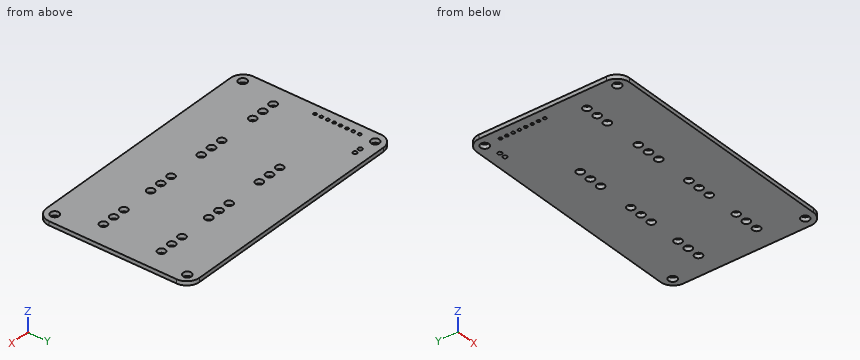
from build123d import *

# Parameters (mm, degrees)
BOSS_EXTRUDE1_DEPTH = 1.6
MULTI_LAYER_R       = 0.6
MULTI_LAYER_R_2     = 1.5
MULTI_LAYER_R_3     = 0.8
MULTI_LAYER_R_4     = 1.6500127
CUT_EXTRUDE2_DEPTH  = 1.6


with BuildPart() as part:
    # BoardOutLine → Boss-Extrude1 (new body)
    with BuildSketch(Plane.XY):
        with BuildLine():
            Line((0, -55), (0, -5))
            ThreePointArc((0, -5), (1.464466094, -1.464466094), (5, 0))
            Line((5, 0), (95, 0))
            ThreePointArc((95, 0), (98.535533906, -1.464466094), (100, -5))
            Line((100, -5), (100, -55))
            ThreePointArc((100, -55), (98.535533906, -58.535533906), (95, -60))
            Line((95, -60), (5, -60))
            ThreePointArc((5, -60), (1.464466094, -58.535533906), (0, -55))
        make_face()
    extrude(amount=BOSS_EXTRUDE1_DEPTH)

    # Multi-Layer → Cut-Extrude2 (cut)
    with BuildSketch(Plane.XY.offset(1.6)):
        with Locations((3.937007874, -25.172974346)):
            Circle(MULTI_LAYER_R)
        with Locations((3.937007874, -22.673101346)):
            Circle(MULTI_LAYER_R)
        with Locations((3.937007874, -20.172974346)):
            Circle(MULTI_LAYER_R)
        with Locations((3.937007874, -17.673101346)):
            Circle(MULTI_LAYER_R)
        with Locations((3.937007874, -15.172974346)):
            Circle(MULTI_LAYER_R)
        with Locations((3.937007874, -12.673101346)):
            Circle(MULTI_LAYER_R)
        with Locations((3.937007874, -10.172974346)):
            Circle(MULTI_LAYER_R)
        with Locations((32.974345949, -41.021082042)):
            Circle(MULTI_LAYER_R_2)
        with Locations((37.973075946, -41.021082042)):
            Circle(MULTI_LAYER_R_2)
        with Locations((42.974345949, -41.021082042)):
            Circle(MULTI_LAYER_R_2)
        with Locations((57.739395479, -41.021082042)):
            Circle(MULTI_LAYER_R_2)
        with Locations((62.738125476, -41.021082042)):
            Circle(MULTI_LAYER_R_2)
        with Locations((67.739395479, -41.021082042)):
            Circle(MULTI_LAYER_R_2)
        with Locations((80.853441707, -41.021082042)):
            Circle(MULTI_LAYER_R_2)
        with Locations((85.852171704, -41.021082042)):
            Circle(MULTI_LAYER_R_2)
        with Locations((90.853441707, -41.021082042)):
            Circle(MULTI_LAYER_R_2)
        with Locations((43.225806452, -18.034036068)):
            Circle(MULTI_LAYER_R_2)
        with Locations((38.227076454, -18.034036068)):
            Circle(MULTI_LAYER_R_2)
        with Locations((33.225806452, -18.034036068)):
            Circle(MULTI_LAYER_R_2)
        with Locations((67.990855982, -18.034036068)):
            Circle(MULTI_LAYER_R_2)
        with Locations((62.992125984, -18.034036068)):
            Circle(MULTI_LAYER_R_2)
        with Locations((57.990855982, -18.034036068)):
            Circle(MULTI_LAYER_R_2)
        with Locations((91.10490221, -18.034036068)):
            Circle(MULTI_LAYER_R_2)
        with Locations((86.106172212, -18.034036068)):
            Circle(MULTI_LAYER_R_2)
        with Locations((81.10490221, -18.034036068)):
            Circle(MULTI_LAYER_R_2)
        with Locations((10.033020066, -5.08001016)):
            Circle(MULTI_LAYER_R_3)
        with Locations((12.573025146, -5.08001016)):
            Circle(MULTI_LAYER_R_3)
        with Locations((7.828295657, -41.021082042)):
            Circle(MULTI_LAYER_R_2)
        with Locations((12.827025654, -41.021082042)):
            Circle(MULTI_LAYER_R_2)
        with Locations((17.828295657, -41.021082042)):
            Circle(MULTI_LAYER_R_2)
        with Locations((3.937007874, -27.673050546)):
            Circle(MULTI_LAYER_R)
        with Locations((4, -4)):
            Circle(MULTI_LAYER_R_4)
        with Locations((96, -56)):
            Circle(MULTI_LAYER_R_4)
        with Locations((96, -4)):
            Circle(MULTI_LAYER_R_4)
        with Locations((4, -56)):
            Circle(MULTI_LAYER_R_4)
    extrude(amount=-CUT_EXTRUDE2_DEPTH, mode=Mode.SUBTRACT)


solid = part.part
Geometry: final body of the model. Coordinates: model frame, mm. Give positions to 0.01 mm unless a question says otherwise; leave off trailing zeros. Loops run counter-clockwise (first coordinate to the right, second up) from the corner with the lowest first, then second, coordinate; pieces in that order, holes last. Notation, with made-up numbers: (-16, 89) - (12, 89) arc R29 ccw to (12, 114) - close; hole circle Ø9 at (64, 17.25). An arc over 180 degrees is marked (long way). One line per question, with ' | ' between items. Start each with the question number.
(1) Section query B-B on z = 1.2. Count the separate pieces of the cut face and the enclosed holes in it, then the cut area to 3 significant figures.
(2) Contact query for a flat-ended pin moving along its axis: pin 1 (1.5 mm diameter, centred on x = 66, y = -35.5, fed in from -Z). Output: stop coordinate, or through.
(3) Ray query, line 1 (Y direction, x = 38, z = 0.3); line 2 (Y direction, x = 44, z = 0.1); line 3 (X direction, y = -13, z = 1.45). Return the intervals inside material, ascending. Write a range as from..to.
(4) Section query A-A on y = -56. Return loops of the section in (x, z), then the cut area to 3 significant figures.
The answers:
1) separate pieces: 1 | enclosed holes: 35 | area: 5,780 mm2
2) pin 1: z = 0
3) line 1: -60..-42.52, -39.52..-19.52, -16.55..0 | line 2: -60..-42.12, -39.93..-19.32, -16.75..0 | line 3: 0..3.43, 4.44..100
4) outline: (0.1, 0) - (2.35, 0) - (2.35, 1.6) - (0.1, 1.6) - close; (5.65, 0) - (94.35, 0) - (94.35, 1.6) - (5.65, 1.6) - close; (97.65, 0) - (99.9, 0) - (99.9, 1.6) - (97.65, 1.6) - close | area: 149 mm2
